```python
from build123d import *

# Parameters (mm, degrees)
F3_DEPTH = 50
F4_DEPTH = 50
F5_DEPTH = 50


with BuildPart() as f3:
    # F0 (on Top) → F3 (new body, symmetric)
    with BuildSketch(Plane.XY):
        with BuildLine():
            Line((21.297112, 15.841494), (38.456534, 31.189908))
            ThreePointArc((38.456534, 31.189908), (-49.496281, -1.35408), (40.104275, -29.040704))
            Line((40.104275, -29.040704), (12.797512, -23.253894))
            ThreePointArc((12.797512, -23.253894), (-25.936908, 5.638858), (21.297112, 15.841494))
        make_face()
    extrude(amount=F3_DEPTH, both=True)

    # F1 (on Front) → F4 (intersect, symmetric)
    with BuildSketch(Plane.XZ):
        Polygon((-20, 50), (-50, 50), (-50, -50), (-20, -50), (50, -50), (50, -24.378916), (-20, -24.378916), (-20, -10.240086), (35, -10.240086), (35, 10.474946), (-20, 10.474946), (-20, 31.586639), (50, 31.586639), (50, 50), align=None)
    extrude(amount=F4_DEPTH, both=True, mode=Mode.INTERSECT)

    # F2 (on Right) → F5 (intersect, symmetric)
    with BuildSketch(Plane.YZ):
        Polygon((49.905006, 26.793262), (49.905006, 50.518591), (-49.905006, 50.518591), (-49.905006, 26.793262), (-49.905006, -50.518591), (-17.180409, -50.518591), (-17.180409, -17.793998), (38.448131, -17.793998), (38.448131, 0), (38.448131, 10.222353), (-17.180409, 10.222353), (-17.180409, 26.793262), align=None)
    extrude(amount=F5_DEPTH, both=True, mode=Mode.INTERSECT)


solid = f3.part
```
For this review, take the finished solid that the model builds, in its own axes (mm). A direction names the side the tool comes from. Round coordinates to 2 decimals unless told otherwise and drop trailing zeros. Write each loop counter-clockwise with the first axis right and the second up, starting at its lowest first coordinate (ties: lowest second). Pieces come first, ordered by that corner, then holes. Notation, with made-up numbers: (89.25, -1.5) -> (102.25, -1.5) arc R14 ccw to (102.25, 13.5) -> close; hole circle Ø2 at (87.5, -6). An arc over 180 degrees is marked (long way). One line per question, with ' | ' between items. Start each with the question number.
(1) Add section D-D, the plane y = 12. Write out the cut boundary in (x, z).
(2) Tool access review of faces 1 (the face through (9, 36, 31.587)), 2 (the face through (-33, -17.18, 18)), 3 (the face through (0, 38.448, -1)): name each direction out of +Z, -Z, +X, -X, +Y, -Y from which nothing blocks a thin tool from reaching the whole face with its end or side.
(3) Add section B-B, the plane x = 17. Write out the cut boundary in (y, z) (3 decimals).
(4) Add section A-A, the plane y = 0. Write out the cut boundary in (x, z), plus the area to 3 significant figures.
(5) Mouldability with a two-part tool opening along Y and no side actions: class faces 4 (the face through (7, 29, -10.24)), 5 (the face through (26.642, -26.188, 40.922)), 6 (the face through (-33, -17.18, -34)) as released by +Y, released by -Y, zero draft, split by the parting line, or undercut.
(6) Add section C-C, the plane x = 0. Write out the cut boundary in (y, z).
(7) For line 1 along Z through (x, y) = (8, 37); line 2 along Y through (x, z) = (0, 10); line 3 along Z through (x, y) = (-22, 17), list the stretches that pass through material, from the lowest coordinate up. Write a range as from..to.
(8) Insertion check: P1, Ø5.5, axis at y = -30, z = 2, coming from the +X side; P2, Ø12, axis at y = 21, z = 28.5, coming from the -X side; P3, Ø1, axis at x = -20.5, z = -25.5, coming from the -Y side. Each pin has a flat end and moves straight along its axis. Give the tip position at first contact, or say it passes through.
Answer list:
1) outline: (-48.04, -17.79) -> (-23.68, -17.79) -> (-23.68, 10.22) -> (-48.04, 10.22) -> close; (-48.04, 26.79) -> (-23.68, 26.79) -> (-23.68, 50) -> (-48.04, 50) -> close
2) face 1: +X, +Y, -Y | face 2: +X, -X, +Y | face 3: -Z, +X, -X, +Y
3) outline: (-46.505, -50) -> (-24.144, -50) -> (-24.144, -24.379) -> (-46.505, -24.379) -> close; (-46.505, -10.24) -> (-24.144, -10.24) -> (-24.144, 10.475) -> (-46.505, 10.475) -> close; (-46.505, 31.587) -> (-24.144, 31.587) -> (-24.144, 50) -> (-46.505, 50) -> close; (20.384, -10.24) -> (38.448, -10.24) -> (38.448, 10.222) -> (20.384, 10.222) -> close; (20.384, 31.587) -> (46.505, 31.587) -> (46.505, 50) -> (20.384, 50) -> close
4) outline: (-49.51, -17.79) -> (-26.54, -17.79) -> (-26.54, 10.22) -> (-49.51, 10.22) -> close; (-49.51, 26.79) -> (-26.54, 26.79) -> (-26.54, 50) -> (-49.51, 50) -> close | area: 1,180 mm²
5) face 4: zero draft | face 5: undercut | face 6: released by +Y
6) outline: (-49.51, -50) -> (-26.54, -50) -> (-26.54, -24.38) -> (-49.51, -24.38) -> close; (-49.51, -10.24) -> (-26.54, -10.24) -> (-26.54, 10.47) -> (-49.51, 10.47) -> close; (-49.51, 31.59) -> (-26.54, 31.59) -> (-26.54, 50) -> (-49.51, 50) -> close; (26.54, -10.24) -> (38.45, -10.24) -> (38.45, 10.22) -> (26.54, 10.22) -> close; (26.54, 31.59) -> (49.51, 31.59) -> (49.51, 50) -> (26.54, 50) -> close
7) line 1: -10.24..10.22, 31.59..50 | line 2: -49.51..-26.54, 26.54..38.45 | line 3: -17.79..10.22, 26.79..50
8) P1: x = 35 | P2: x = -47.19 | P3: y = -45.3
